Could you check a few things on this drawing? It's one solid part, dimensions in mm from its lowest x, y, z. A direction names the side the tool comes from. Give positions to 0.01 mm unless a question says otherwise; leave off trailing zeros. Order: outer loops, then holes, each group sorted by start corner. A loop starts at its lowest first (then second) coordinate and runs counter-clockwise, first axis right, second up.
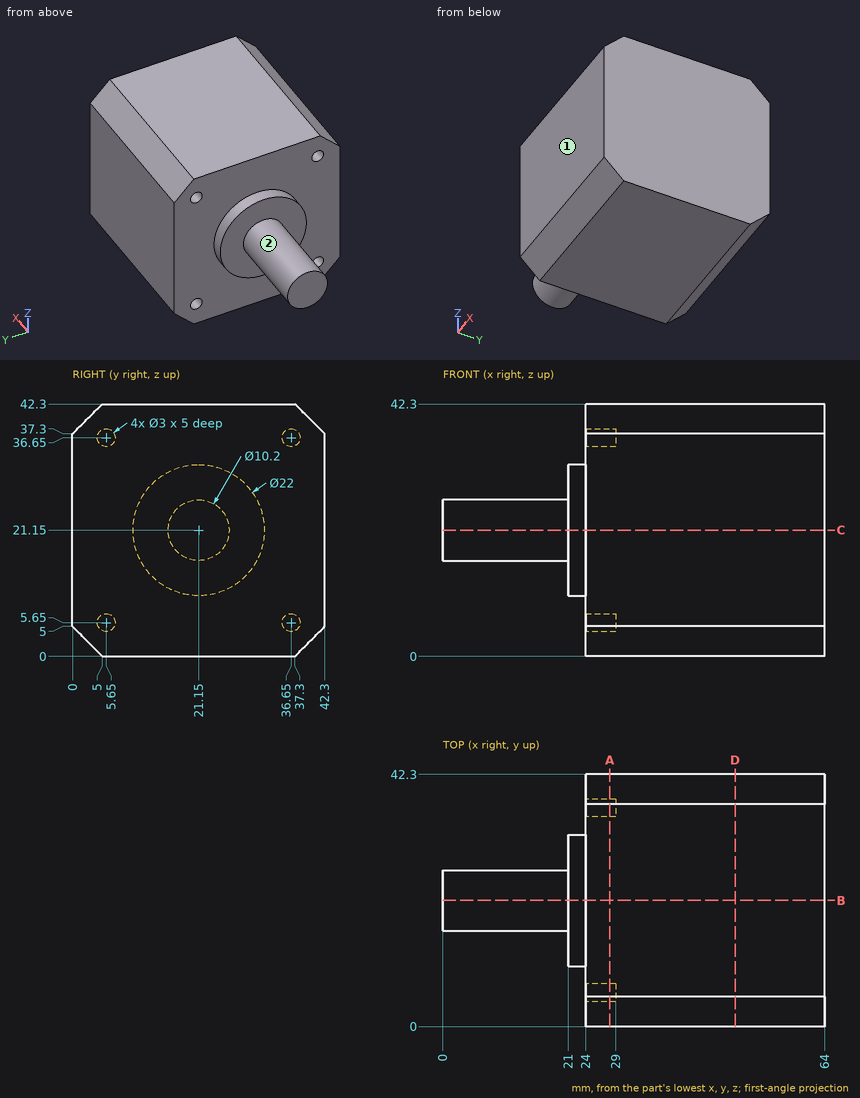
1) If I drill on line 1 (Y direction, x = 25.35, z = 5.65); line 2 (Y direction, x = 24.5, z = 37.5); line 3 (Z direction, x = 25, y = 5), over which ranges is the centre line in solid material (lowest first)?
2) Suppose I cut it at D-D (x = 49). Please give me the cut outline in (y, z), and give its area (3 significant figures).
3) I'm going to push flat-ended pins straight in: pin 1 Ø1 at (y, z) = (24.5, 12) entering from -X; pin 2 Ø1.5 at (y, z) = (5, 5.5) entering from -X; pin 3 Ø3.5 at (y, z) = (36, 6) entering from -X. Where does each tip first touch, or does it pass through?
4) Suppose I cut it at A-A (x = 28). Please give me the cut outline in (y, z), and give its area (3 significant figures).
5) Suppose I cut it at B-B (y = 21.15). Please give me the cut outline in (x, z), and give its area (3 significant figures).
6) Which directions (+Z, -Z, +X, -X, +Y, -Y) give clear straight access to the entire face, cutting with the end or side of a thin tool? Please do the marked faces 1 and 2.
Results:
1. line 1: y = 0 to 4.15, 7.15 to 35.15, 38.15 to 42.3
1. line 2: y = 0.2 to 4.41, 6.89 to 35.41, 37.89 to 42.1
1. line 3: z = 0 to 4.3, 7 to 35.3, 38 to 42.3
2. outline: (0, 5) - (5, 0) - (37.3, 0) - (42.3, 5) - (42.3, 37.3) - (37.3, 42.3) - (5, 42.3) - (0, 37.3) - close
2. area: 1,740 mm2
3. pin 1: stops at x = 21
3. pin 2: stops at x = 29
3. pin 3: stops at x = 24
4. outline: (0, 5) - (5, 0) - (37.3, 0) - (42.3, 5) - (42.3, 37.3) - (37.3, 42.3) - (5, 42.3) - (0, 37.3) - close; hole circle Ø3 at (5.65, 5.65); hole circle Ø3 at (5.65, 36.65); hole circle Ø3 at (36.65, 5.65); hole circle Ø3 at (36.65, 36.65)
4. area: 1,710 mm2
5. outline: (0, 16.05) - (21, 16.05) - (21, 10.15) - (24, 10.15) - (24, 0) - (64, 0) - (64, 42.3) - (24, 42.3) - (24, 32.15) - (21, 32.15) - (21, 26.25) - (0, 26.25) - close
5. area: 1,970 mm2
6. face 1: +Z, -Z, +X, -X, -Y
6. face 2: -X
